```python
from build123d import *

# Parameters (mm, degrees)
BOSS_EXTRUDE2_DEPTH = 15
SKETCH4_R           = 3
CUT_EXTRUDE2_DEPTH  = 34.634060118
SKETCH7_R           = 3
CUT_EXTRUDE4_DEPTH  = 34.634060118


with BuildPart() as part:
    # Sketch3 → Boss-Extrude2 (new body)
    with BuildSketch(Plane(origin=(0, 0, 0), x_dir=(1, 0, 0), z_dir=(0, 1, 0))):
        Polygon((0, 0), (22.5, 0), (22.5, 22.5), (20, 22.5), (20, 2.5), (0, 2.5), align=None)
    extrude(amount=BOSS_EXTRUDE2_DEPTH)

    # Sketch4 → Cut-Extrude2 (cut, through all)
    with BuildSketch(Plane(origin=(0, 0, -2.5), x_dir=(-1, 0, 0), z_dir=(0, 0, -1))):
        with Locations((-10, 7.5)):
            Circle(SKETCH4_R)
    extrude(amount=-CUT_EXTRUDE2_DEPTH, mode=Mode.SUBTRACT)

    # Sketch7 → Cut-Extrude4 (cut, through all)
    with BuildSketch(Plane.ZY.offset(-20)):
        with Locations((-17.5, 7.5)):
            Circle(SKETCH7_R)
    extrude(amount=-CUT_EXTRUDE4_DEPTH, mode=Mode.SUBTRACT)


solid = part.part
```
For this review, take the finished solid that the model builds, in its own axes (mm). A direction names the side the tool comes from. Round coordinates to 2 decimals unless told otherwise and drop trailing zeros. Write each loop counter-clockwise with the first axis right and the second up, starting at its lowest first coordinate (ties: lowest second). Pieces come first, ordered by that corner, then holes. Notation, with made-up numbers: (18.25, 69.5) - (63.25, 69.5) arc R36 cw to (63.25, 105.5) - close; hole circle Ø10 at (-39.5, 79.25). An arc over 180 degrees is marked (long way). Answer as CSV lines item,"result". Start each with the question number.
(1) Mouldability with a two-part tool opening along Y and no side actions: class faces 1 (the flat face through (14, 7, 0)), 2 (the cylindrical face through (12.4, 5.7, -1.3)), 3 (the flat face through (16, 0, -2)) as +Y half, -Y half, draft (parallel to the pull), parting line (faces both ways), or undercut.
(2) Add section C-C, the plane x = 10. State the section outline as (y, z) points, plus the area to 3 significant figures.
(3) Add section D-D, the plane y = 13. State the section outline as (x, z) points.
(4) Machinability: for faces 4 (the cylindrical face through (21.2, 7.6, -20.5)), 5 (the flat face through (10, 4, -2.5)), which of the approach directions +Z, -Z, +X, -X, +Y, -Y give a long, thin tool a straight path to every point of the face, cutting with its end or side? Answer none if there is none.
(5) For pin 1 (8 mm diameter, centred on y = 7.5, z = -17.5, fed in from -X); pin 2 (5 mm diameter, centred on x = 7, y = 13, fed in from -Z), all flat-tipped, find the tip position at first contact; note any pin that passes through.
(6) Add section A-A, the plane z = -17.5. State the section outline as (x, y) points, plus the area to 3 significant figures.
(7) Add section B-B, the plane y = 7.5. State the section outline as (x, z) points.
(8) For line 1 (Y direction, x = 10, z = -1); line 2 (Z direction, x = 4, y = 9.5); line 3 (X direction, y = 9.5, z = -9.25), list the stretches that pass through material, from the lowest coordinate up.
From the geometry:
1,face 1,"draft"
1,face 2,"undercut"
1,face 3,"-Y half"
2,outline,"(0, -2.5) - (4.5, -2.5) - (4.5, 0) - (0, 0) - close; (10.5, -2.5) - (15, -2.5) - (15, 0) - (10.5, 0) - close"
2,area,"22.5 mm²"
3,outline,"(0, -2.5) - (20, -2.5) - (20, -22.5) - (22.5, -22.5) - (22.5, 0) - (0, 0) - close"
4,face 4,"+X, -X"
4,face 5,"-Z, -X, +Y, -Y"
5,pin 1,"stops at x = 20"
5,pin 2,"stops at z = -2.5"
6,outline,"(20, 0) - (22.5, 0) - (22.5, 4.5) - (20, 4.5) - close; (20, 10.5) - (22.5, 10.5) - (22.5, 15) - (20, 15) - close"
6,area,"22.5 mm²"
7,outline,"(0, -2.5) - (7, -2.5) - (7, 0) - (0, 0) - close; (13, -2.5) - (20, -2.5) - (20, -14.5) - (22.5, -14.5) - (22.5, 0) - (13, 0) - close; (20, -22.5) - (22.5, -22.5) - (22.5, -20.5) - (20, -20.5) - close"
8,line 1,"y = 0 to 4.5, 10.5 to 15"
8,line 2,"z = -2.5 to 0"
8,line 3,"x = 20 to 22.5"
